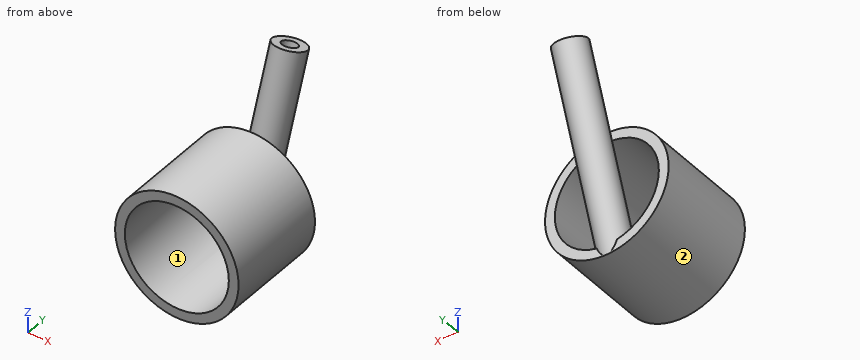
from build123d import *

# Parameters (mm, degrees)
SKETCH1_R           = 13.2715
SKETCH1_R_2         = 11.176
BOSS_EXTRUDE1_DEPTH = 22.225
SKETCH2_R           = 3.429
SKETCH2_R_2         = 1.651
BOSS_EXTRUDE2_DEPTH = 40.64


with BuildPart() as part:
    # Sketch1 → Boss-Extrude1 (new body)
    with BuildSketch(Plane(origin=(0, 0, 0), x_dir=(1, 0, 0), z_dir=(0, 1, 0))):
        Circle(SKETCH1_R)
        Circle(SKETCH1_R_2, mode=Mode.SUBTRACT)
    extrude(amount=BOSS_EXTRUDE1_DEPTH)

    # Sketch2 → Boss-Extrude2 (add)
    with BuildSketch(Plane(origin=(0, -1.665546755, -4.576052101), x_dir=(-1, 0, 0), z_dir=(0, -0.342020143, -0.939692621))):
        with Locations((0, 21.994788829)):
            Circle(SKETCH2_R)
        with Locations((0, 21.994788829)):
            Circle(SKETCH2_R_2, mode=Mode.SUBTRACT)
    extrude(amount=-BOSS_EXTRUDE2_DEPTH)


solid = part.part
Here's how the part is built. I have some questions about the finished solid (model axes, mm). Face numbers are marked on the shaded views. Round coordinates to 2 decimals unless told otherwise and drop trailing zeros. Write each loop counter-clockwise with the first axis right and the second up, starting at its lowest first coordinate (ties: lowest second). Pieces come first, ordered by that corner, then holes.
1. I need wall thicknesses on L1, parallel to X at y = 17, z = 0; L2, parallel to X at y = 18.5, z = -8.5. Which ranges of each line are inside material? Lowest first, please.
2. Suppose I cut it at A-A (x = -7). List the corners of the cut face in (y, z) for me (3 decimals).
3. Suppose I cut it at C-C (z = 1.5). State how many separate pieces and enclosed holes the cut face has, and give its area (3 significant figures).
4. Suppose I cut it at D-D (x = 6.5). List the corners of the cut face in (y, z) for me (3 decimals).
5. Suppose I cut it at B-B (y = 10). List the corners of the cut face in (x, z) for me.
6. If we mould it in two halves opening along Z, with no side actions, what happens to the marked faces 1 and 2? For each: released by +Z, released by -Z, zero draft, split by the parting line, or undercut.
7. Will these pins go through, and if not, where does the flat tip stop? pin 1 Ø4 at (y, z) = (24.5, 20.5) entering from +X; pin 2 Ø4 at (x, y) = (-3.5, 18) entering from -Z; pin 3 Ø1 at (x, z) = (-1, -8.5) entering from +Y; pin 4 Ø5 at (x, y) = (-9, 19) entering from +Z.
Answer sheet:
1. L1: x = -13.27 to -11.18, 11.18 to 13.27
1. L2: x = -10.19 to -7.26, -2.98 to 2.98, 7.26 to 10.19
2. outline: (0, -11.275) - (22.225, -11.275) - (22.225, -8.712) - (0, -8.712) - close; (0, 8.712) - (22.225, 8.712) - (22.225, 11.275) - (0, 11.275) - close
3. separate pieces: 3
3. enclosed holes: 1
3. area: 124 mm2
4. outline: (0, -11.571) - (22.225, -11.571) - (22.225, -9.091) - (0, -9.091) - close; (0, 9.091) - (22.225, 9.091) - (22.225, 11.571) - (0, 11.571) - close
5. outline: circle Ø26.54 at (0, 0); hole circle Ø22.35 at (0, 0)
6. face 1: undercut
6. face 2: split by the parting line
7. pin 1: passes through
7. pin 2: stops at z = -13.19
7. pin 3: stops at y = 24.03
7. pin 4: stops at z = 11.57
